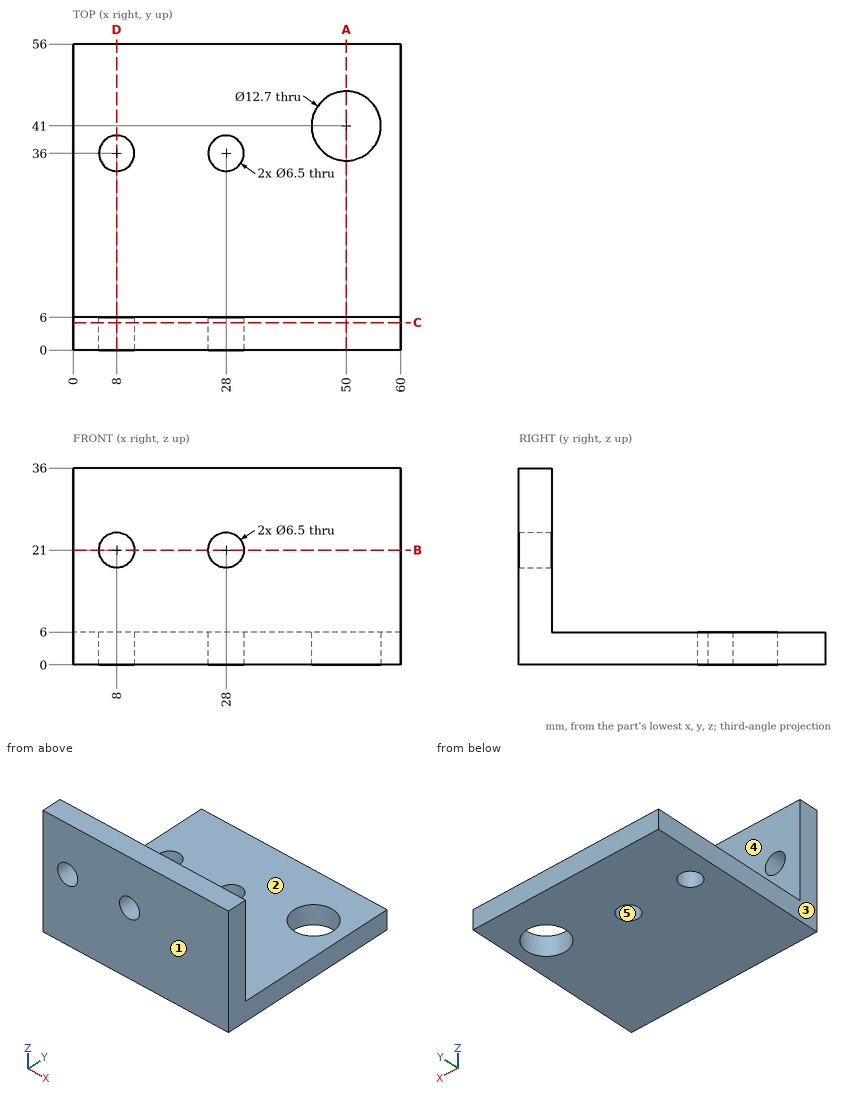
Can you work these out from the drawing? Everything is in mm from the part's minimum corner. A direction names the side the tool comes from. Give positions to 0.01 mm unless a question says otherwise; leave off trailing zeros. Loops run counter-clockwise (first coordinate to the right, second up) from the corner with the lowest first, then second, coordinate; pieces in that order, holes last. Notation, with made-up numbers: (4, 10) -> (62, 10) arc R31 cw to (62, 39) -> close; hole circle Ø5 at (55.5, -39.75). An arc over 180 degrees is marked (long way). Write item = value, one per line.
1) Suppose I cut it at A-A on x = 50. Write out the boundary of the cut face in (y, z).
Check result:
outline = (0, 0) -> (34.65, 0) -> (34.65, 6) -> (6, 6) -> (6, 36) -> (0, 36) -> close; (47.35, 0) -> (56, 0) -> (56, 6) -> (47.35, 6) -> close
2) Thinking about a two-plate mould opening in Y: for the marked faces 3, 4 and 5, which applies, released by +Y, released by -Y, zero draft, split by the parting line, or undercut?
Check result:
face_3 = zero draft
face_4 = released by +Y
face_5 = undercut
3) Suppose I cut it at D-D on x = 8. Write out the boundary of the cut face in (y, z).
Check result:
outline = (0, 0) -> (32.75, 0) -> (32.75, 6) -> (6, 6) -> (6, 17.75) -> (0, 17.75) -> close; (0, 24.25) -> (6, 24.25) -> (6, 36) -> (0, 36) -> close; (39.25, 0) -> (56, 0) -> (56, 6) -> (39.25, 6) -> close
4) I need wall thicknesses on L1, parallel to X at y = 1.75, z = 21; L2, parallel to Z at x = 8, y = 1.7; L3, parallel to Y at x = 28, z = 1. Which ranges of each line are inside material? Lowest first, please. Write a range as from..to.
Check result:
L1 = 0..4.75, 11.25..24.75, 31.25..60
L2 = 0..17.75, 24.25..36
L3 = 0..32.75, 39.25..56
5) For the marked faces 1 and 2, which set-ups out of +Z, -Z, +X, -X, +Y, -Y let a thin tool reach every point of the face, with its end or its side?
Check result:
face_1 = +Z, -Z, +X, -X, -Y
face_2 = +Z, +X, -X, +Y
6) Suppose I cut it at C-C on y = 5. Write out the boundary of the cut face in (x, z).
Check result:
outline = (0, 0) -> (60, 0) -> (60, 36) -> (0, 36) -> close; hole circle Ø6.5 at (8, 21); hole circle Ø6.5 at (28, 21)
7) Will these pins go through, and if not, where does the flat tip stop? pin 1 (15 mm diameter, centred on x = 24, y = 36.5, fed in from +Z); pin 2 (1.5 mm diameter, centred on x = 10, z = 17, fed in from +Y).
Check result:
pin_1 = 6
pin_2 = 6
8) Suppose I cut it at B-B on z = 21. Write out the boundary of the cut face in (x, y), then the cut area to 3 significant figures.
Check result:
outline = (0, 0) -> (4.75, 0) -> (4.75, 6) -> (0, 6) -> close; (11.25, 0) -> (24.75, 0) -> (24.75, 6) -> (11.25, 6) -> close; (31.25, 0) -> (60, 0) -> (60, 6) -> (31.25, 6) -> close
area = 282 mm2
